Design review of the part built by this model. Coordinates are the model's own, in mm. Round coordinates to 2 decimals unless told otherwise and drop trailing zeros. Loops run counter-clockwise (first coordinate to the right, second up) from the corner with the lowest first, then second, coordinate; pieces in that order, holes last. Notation, with made-up numbers: (-34, 2.5) -> (-2, 2.5) arc R11 ccw to (-2, 9.5) -> close; hole circle Ø8 at (56, 65). An arc over 180 degrees is marked (long way). Answer as CSV lines item,"result". Start each with the question number.
(1) Take a section at A-A, the plane x = 0. Write out the cut boundary in (y, z), and give its area (3 significant figures).
(2) Take a section at B-B, the plane y = -256.5. Write out the cut boundary in (x, z), and give its area (3 significant figures).
(3) To check wall thickness, follow line 1 (Y direction, x = 0, z = 11); line 2 (Y direction, x = 163, z = 16); line 3 (X direction, y = -218.5, z = 18.5). State the ranges of each line that lie inside material, in increasing order. Write a range as from..to.
(4) For P1, Ø1.5, axis at x = -142.5, z = 30.5, coming from the +Y side; P2, Ø2, axis at x = 131.5, z = 34, coming from the -Y side; P3, Ø6, axis at x = -77.5, z = 9.5, coming from the -Y side, all flat-tipped, find the tip position at first contact; note any pin that passes through.
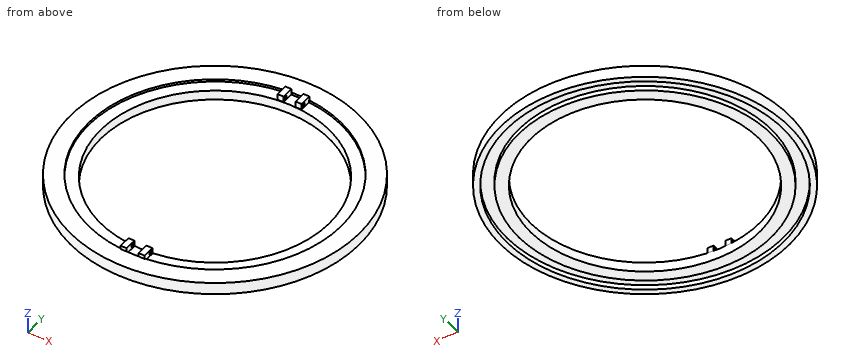
Autodesk Inventor part; units mm, degrees
ref_plane "YZ Plane" through (0, 0, 0) normal (1, 0, 0) x (0, 1, 0)
ref_plane "XZ Plane" through (0, 0, 0) normal (0, 1, 0) x (-1, 0, 0)
ref_plane "XY Plane" through (0, 0, 0) normal (0, 0, 1) x (1, 0, 0)
sketch "Sketch1" plane through (0, 0, 0) normal (0, 0, 1) x (1, 0, 0)
  circle A0 centre (0, 0) radius 600
  circle A1 centre (0, 0) radius 575
  circle A2 centre (0, 0) radius 525
  circle A3 centre (0, 0) radius 475
  dimension "d2" = 1200
  dimension "d1" = 1150
  dimension "d0" = 1050
  dimension "d9" = 950
extrude "Extrusion1" add sketch "Sketch1" along normal blind 50 contours A0 | A1 | A2 | A3
extrude "Extrusion2" cut sketch "Sketch1" along normal blind 20 contours A1
extrude "Extrusion3" cut sketch "Sketch1" along normal blind 315.5 contours A3
sketch "Sketch3" plane through (0, 0, 0) normal (0, 0, 1) x (1, 0, 0)
  circle A0 centre (0, 0) radius 475
  line L0 (475, 0) -> (525, 0)
  circle A1 centre (0, 0) radius 525
  line L1 (500, 0) -> (500, 50)
  line L2 (500, 50) -> (430, 50)
  line L3 (430, 50) -> (430, -50)
  line L4 (430, -50) -> (500, -50)
  line L5 (500, -50) -> (500, 50)
  line L6 (0, -117.9134) -> (0, 153.6807)
  line L7 (-500, 50) -> (-430, 50)
  line L8 (-430, 50) -> (-430, -50)
  line L9 (-430, -50) -> (-500, -50)
  line L10 (-500, -50) -> (-500, 50)
  line L11 (465, 0) -> (465, 25)
  line L12 (465, 25) -> (-465, 25)
  line L13 (-465, 25) -> (-465, -25)
  line L14 (-465, -25) -> (465, -25)
  line L15 (465, -25) -> (465, 25)
  point P0 (472.3611, -50)
  point P1 (472.3611, 50)
  point P2 (430, -25)
  point P3 (430, 25)
  point P4 (-430, -25)
  point P5 (-430, 25)
  dimension "d12" = 50
  dimension "d13" = 70
  dimension "d14" = 100
  dimension "d17" = 50
extrude "Extrusion4" [suppressed]
sketch "Sketch4" plane through (-472.3611, 50, 0) normal (0, 1, 0) x (1, 0, 0)
  line L0 (42.3611, 0) -> (42.3611, -50)
  line L1 (42.3611, -50) -> (24.8611, -50) construction
  line L2 (42.3611, -50) -> (0, -50)
  line L3 (24.8611, -50) -> (24.8611, -25) construction
  line L4 (42.3611, 0) -> (0, 0)
  line L5 (24.8611, -50) -> (49.8611, -50) construction
  circle A0 centre (24.8611, -25) radius 7.9375
  point P0 (472.3611, 0)
  dimension "d18" = 17.5
  dimension "d19" = 25
  dimension "d20" = 90
  dimension "d21" = 15.875
extrude "Extrusion5" [suppressed]
sketch "Sketch5" plane through (430, 50, 0) normal (0, 1, 0) x (1, 0, 0)
  line L0 (42.3611, -50) -> (0, -50)
  line L1 (0, -50) -> (0, -25) construction
  line L2 (0, 0) -> (0, -50)
  line L3 (42.3611, 0) -> (42.3611, -50)
  line L4 (0, -25) -> (21.1805, -25) construction
  circle A0 centre (21.1805, -25) radius 7.9375
  point P0 (-430, 0)
  dimension "d25" = 21.1806
  dimension "d26" = 15.875
extrude "Extrusion6" [suppressed]
sketch "Sketch6" plane through (0, 0, 50) normal (0, 0, 1) x (1, 0, 0)
  circle A0 centre (0, 0) radius 525
extrude "Extrusion7" cut sketch "Sketch6" against normal blind 10
sketch "Sketch7" plane through (0, 0, 40) normal (0, 0, 1) x (1, 0, 0)
  circle A0 centre (0, 0) radius 475
  circle A1 centre (0, 0) radius 600
  line L0 (0, 475) -> (-290.4738, 475)
  line L1 (-290.4738, 475) -> (-290.4738, 525)
  line L2 (-290.4738, 525) -> (0, 525)
  line L3 (0, 525) -> (0, 475)
  line L4 (0, 475) -> (291, 475)
  line L5 (291, 475) -> (291, 525)
  line L6 (291, 525) -> (0, 525)
  line L7 (0, 525) -> (0, 475)
  line L8 (0, 475) -> (25, 475)
  line L9 (25, 475) -> (0, 475)
  line L10 (0, 475) -> (-25, 475)
  line L11 (-50, 475) -> (-25, 475)
  line L12 (-25, 475) -> (-25, 525)
  line L13 (-25, 525) -> (-50, 525)
  line L14 (-50, 525) -> (-50, 475)
  line L15 (25, 475) -> (50, 475)
  line L16 (50, 475) -> (50, 525)
  line L17 (50, 525) -> (25, 525)
  line L18 (25, 525) -> (25, 475)
  dimension "d31" = 50
  dimension "d32" = 50
  dimension "d33" = 25
  dimension "d34" = 25
  dimension "d35" = 25
  dimension "d36" = 25
  dimension "d37" = 50
  dimension "d38" = 25
  dimension "d39" = 50
extrude "Extrusion8" add sketch "Sketch7" along normal blind 25 contours L0 L14 L2 L12 | L18 L6 L16 L4
sketch "Sketch8" plane through (-25, 475, 40) normal (1, 0, 0) x (0, 0, -1)
  line L0 (-25, 0) -> (-12.5, 0) construction
  line L1 (-12.5, 0) -> (-12.5, 12.5) construction
  circle A0 centre (-12.5, 12.5) radius 7.9375
  point P0 (40, -475)
  dimension "d42" = 12.5
  dimension "d43" = 12.5
  dimension "d44" = 15.875
extrude "Extrusion9" cut sketch "Sketch8" along normal blind 75 and the other way blind 25
mirror "Mirror1" about plane through (0, 0, 0) normal (0, 1, 0) of "Extrusion8"
sketch "Sketch9" plane through (-50, -525, 65) normal (-1, 0, 0) x (0, 0, 1)
  line L0 (-25, 50) -> (0, 50)
  line L1 (0, 50) -> (-12.5, 50) construction
  line L2 (-12.5, 50) -> (-12.5, 37.5) construction
  line L3 (-25, 50) -> (-25, 0.5956)
  line L4 (-12.5, 50) -> (0, 50) construction
  circle A0 centre (-12.5, 37.5) radius 7.9375
  point P0 (-65, 525)
  dimension "d49" = 12.5
  dimension "d50" = 90
  dimension "d51" = 15.875
extrude "Extrusion10" cut sketch "Sketch9" against normal up to surface (100 mm away)
properties part number "Top opening"
The answers:
1,outline,"(-600, 0) -> (-575, 0) -> (-575, 20) -> (-525, 20) -> (-525, 0) -> (-475, 0) -> (-475, 40) -> (-525, 40) -> (-525, 50) -> (-600, 50) -> close; (475, 0) -> (525, 0) -> (525, 20) -> (575, 20) -> (575, 0) -> (600, 0) -> (600, 50) -> (525, 50) -> (525, 40) -> (475, 40) -> close"
1,area,"9,500 mm²"
2,outline,"(-542.41, 0) -> (-514.62, 0) -> (-514.62, 20) -> (-458.08, 20) -> (-458.08, 0) -> (-399.79, 0) -> (-399.79, 40) -> (-458.08, 40) -> (-458.08, 50) -> (-542.41, 50) -> close; (399.79, 0) -> (458.08, 0) -> (458.08, 20) -> (514.62, 20) -> (514.62, 0) -> (542.41, 0) -> (542.41, 50) -> (458.08, 50) -> (458.08, 40) -> (399.79, 40) -> close"
2,area,"10,800 mm²"
3,line 1,"-600..-575, -525..-475, 475..525, 575..600"
3,line 2,"-577.43..-551.41, -499.06..-446.16, 446.16..499.06, 551.41..577.43"
3,line 3,"-558.8..-531.87, -477.37..-421.76, 421.76..477.37, 531.87..558.8"
4,P1,"y = 583.02"
4,P2,"y = -585.64"
4,P3,"y = -595.36"
